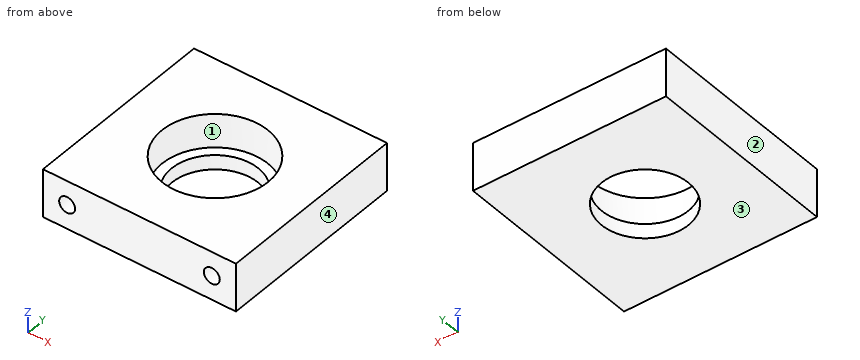
from build123d import *

# Parameters (mm, degrees)
BASE_EXTRUSION_DEPTH       = 10
ESQUISSE2_R                = 11
ENL_V_MAT_EXTRU_1_DEPTH    = 7
ESQUISSE3_R                = 9
ENL_V_MAT_EXTRU_2_DEPTH    = 44.588989435
ESQUISSE4_OUTSIDE_W        = 77.748
ESQUISSE4_OUTSIDE_H        = 67.748
ESQUISSE4_OUTSIDE_W_2      = 40
ESQUISSE4_OUTSIDE_H_2      = 40
ENL_V_MAT_EXTRU_3_DEPTH    = 44.588989435
R_P_TITION_LIN_AIRE1_COUNT = 2
R_P_TITION_LIN_AIRE1_PITCH = 30


with BuildPart() as part:
    # Esquisse1 → Base-Extrusion (new body)
    with BuildSketch(Plane.XY):
        with BuildLine():
            Line((-22.360679775, -20), (22.360679775, -20))
            ThreePointArc((22.360679775, -20), (0, 30), (-22.360679775, -20))
        make_face()
    extrude(amount=BASE_EXTRUSION_DEPTH)

    # Esquisse2 → Enlèv. mat.-Extru.1 (cut)
    with BuildSketch(Plane.XY.offset(10)):
        Circle(ESQUISSE2_R)
    extrude(amount=-ENL_V_MAT_EXTRU_1_DEPTH, mode=Mode.SUBTRACT)

    # Esquisse3 → Enlèv. mat.-Extru.2 (cut, through all)
    with BuildSketch(Plane(origin=(0, 0, 0), x_dir=(-1, 0, 0), z_dir=(0, 0, -1))):
        Circle(ESQUISSE3_R)
    extrude(amount=-ENL_V_MAT_EXTRU_2_DEPTH, mode=Mode.SUBTRACT)

    # Esquisse4 outside → Enlèv. mat.-Extru.3 (cut, through all)
    with BuildSketch(Plane.XY.offset(10)):
        with Locations((0, 5)):
            Rectangle(ESQUISSE4_OUTSIDE_W, ESQUISSE4_OUTSIDE_H)
        Rectangle(ESQUISSE4_OUTSIDE_W_2, ESQUISSE4_OUTSIDE_H_2, mode=Mode.SUBTRACT)
    extrude(amount=-ENL_V_MAT_EXTRU_3_DEPTH, mode=Mode.SUBTRACT)

    # Esquisse5 → Perçage1 (revolve, cut)
    with BuildSketch(Plane(origin=(15, -20, 5), x_dir=(0, 0, -1), z_dir=(1, 0, 0))):
        Polygon((0, 0), (0, 30.991420021), (1.65, 30), (1.65, 0), align=None)
    per_age1 = revolve(axis=Axis((15, -26.35, 5), (0, 1, 0)), mode=Mode.SUBTRACT)

    # Répétition linéaire1: Perçage1 ×2
    with Locations(*[(-i * R_P_TITION_LIN_AIRE1_PITCH, 0, 0) for i in range(1, R_P_TITION_LIN_AIRE1_COUNT)]):
        add(per_age1, mode=Mode.SUBTRACT)


solid = part.part
Input: part model. Units: mm. Frame: model coordinates. Face numbers are marked on the shaded views. Coordinates: 2 decimals unless noted, no trailing zeros. Order: outer loops, then holes, each group sorted by start corner. A loop starts at its lowest first (then second) coordinate and runs counter-clockwise, first axis right, second up. Notation, with made-up numbers: M 28,-15.75 L 87,-15.75 A38 cw 87,23.25 Z; hole C 12,17 d5. An arc over 180 degrees is marked long. Write item = value, one per line. Start each with the question number.
(1) Section B-B on y = 5. Output: boundary loops of the cut face in (x, z), and give its area (3 significant figures).
(2) Pull-direction query (X, two-part tool) for the marked faces 1, 2, 3 and 4; classes: released by +X, released by -X, zero draft, split by the parting line, or undercut.
(3) First-contact query: P1, Ø24, axis at x = 5, y = 1, coming from the +Z side; P2, Ø2, axis at x = 15, z = 5, coming from the -Y side; P3, Ø1.5, axis at x = -4, y = 7, coming from the -Z side. Flat tips, straight axial feed; report the tip coordinate or a pass-through.
(4) Section A-A on x = 0. Output: boundary loops of the cut face in (y, z), and give its area (3 significant figures).
(5) Section C-C on y = -13.5. Output: boundary loops of the cut face in (x, z), and give its area (3 significant figures).
(6) Section D-D on z = 2. Output: boundary loops of the cut face in (x, y), and give its area (3 significant figures).
(7) Line query: line 1 along X through (y, z) = (-11.5, 5); line 2 along Z through (x, y) = (-15, 3); line 3 along Y through (x, z) = (0, 2.1). Output: solid intervals per line, ascending. Write a range as [from, to].
Result set:
q1.outline = M -20,0 L -7.48,0 L -7.48,3 L -9.8,3 L -9.8,10 L -20,10 Z; M 7.48,0 L 20,0 L 20,10 L 9.8,10 L 9.8,3 L 7.48,3 Z; hole C -15,5 d3.3; hole C 15,5 d3.3
q1.area = 201 mm²
q2.face_1 = undercut
q2.face_2 = released by -X
q2.face_3 = zero draft
q2.face_4 = released by +X
q3.P1 = 10
q3.P2 = 10.39
q3.P3 = through
q4.outline = M -20,0 L -9,0 L -9,3 L -11,3 L -11,10 L -20,10 Z; M 9,0 L 20,0 L 20,10 L 11,10 L 11,3 L 9,3 Z
q4.area = 192 mm²
q5.outline = M -20,0 L 20,0 L 20,10 L -20,10 Z; hole C -15,5 d3.3; hole C 15,5 d3.3
q5.area = 383 mm²
q6.outline = M -20,-20 L 20,-20 L 20,20 L -20,20 Z; hole C 0,0 d18
q6.area = 1,350 mm²
q7.line_1 = [-20, -16.65], [-13.35, 13.35], [16.65, 20]
q7.line_2 = [0, 3.35], [6.65, 10]
q7.line_3 = [-20, -9], [9, 20]
